Geometry check sheet. Reference: the model listing, model coordinates, mm. Coordinates: 2 decimals unless noted, no trailing zeros. Write each loop counter-clockwise with the first axis right and the second up, starting at its lowest first coordinate (ties: lowest second). Pieces come first, ordered by that corner, then holes. Notation, with made-up numbers: (52.25, 85.5) -> (81.25, 85.5) arc R30 cw to (81.25, 109.5) -> close; hole circle Ø8 at (51, 51.5). An arc over 180 degrees is marked (long way). Answer in a Markdown table with one row per item. Add a question column.
1. Cross-section at A-A on x = -18. Record the cut outline in (y, z).
2. Cross-section at C-C on y = 0.85. Record the cut outline in (x, z).
3. Scan lines: L1, parallel to X at y = 1.95, z = 43; L2, parallel to Z at x = -31.5, y = 1.7. Record each from-to range of solid material in increasing order. Write a range as from..to.
4. Cross-section at B-B on z = 13. Record the cut outline in (x, y).
```python
from build123d import *

# Parameters (mm, degrees)
F0_W     = 195
F0_H     = 150
F0_W_2   = 172
F0_H_2   = 132
F1_DEPTH = 3
F2_R     = 2.5


with BuildPart() as f1:
    # F0 (on Front) → F1 (new body)
    with BuildSketch(Plane.XZ):
        Rectangle(F0_W, F0_H)
        Rectangle(F0_W_2, F0_H_2, mode=Mode.SUBTRACT)
    extrude(amount=-F1_DEPTH)

    # F2
    f2_edges = [f1.edges().sort_by_distance(p)[0] for p in [
        (-86, 1.5, -66),
        (86, 1.5, -66),
        (86, 1.5, 66),
        (-86, 1.5, 66),
    ]]
    fillet(f2_edges, radius=F2_R)


solid = f1.part
```
Results found:
| question | item | result |
|---|---|---|
| 1 | outline | (0, -75) -> (3, -75) -> (3, -66) -> (0, -66) -> close; (0, 66) -> (3, 66) -> (3, 75) -> (0, 75) -> close |
| 2 | outline | (-97.5, -75) -> (97.5, -75) -> (97.5, 75) -> (-97.5, 75) -> close; hole (-86, -63.5) arc R2.5 ccw to (-83.5, -66) -> (83.5, -66) arc R2.5 ccw to (86, -63.5) -> (86, 63.5) arc R2.5 ccw to (83.5, 66) -> (-83.5, 66) arc R2.5 ccw to (-86, 63.5) -> close |
| 3 | L1 | x = -97.5..-86, 86..97.5 |
| 3 | L2 | z = -75..-66, 66..75 |
| 4 | outline | (-97.5, 0) -> (-86, 0) -> (-86, 3) -> (-97.5, 3) -> close; (86, 0) -> (97.5, 0) -> (97.5, 3) -> (86, 3) -> close |
